Check sheet for the modelled part. Datum: model origin and axes. Units: mm. Face numbers are marked on the shaded views. A direction names the side the tool comes from. Round coordinates to 2 decimals unless told otherwise and drop trailing zeros. Order: outer loops, then holes, each group sorted by start corner. A loop starts at its lowest first (then second) coordinate and runs counter-clockwise, first axis right, second up.
```python
from build123d import *

# Parameters (mm, degrees)
BOSS_EXTRUDE1_DEPTH  = 4.5
SKETCH2_W            = 1
SKETCH2_H            = 6
BOSS_EXTRUDE2_DEPTH  = 2
SKETCH3_R            = 1
SKETCH3_R_2          = 0.5
CUT_EXTRUDE1_DEPTH   = 2
SKETCH3_2_R          = 0.5
BOSS_EXTRUDE3_DEPTH  = 2
FILLET1_R            = 1
SKETCH4_W            = 2.5
SKETCH4_H            = 2.5
CUT_EXTRUDE2_DEPTH   = 5.5000001
FILLET2_R            = 0.3
BOSS_EXTRUDE4_DEPTH  = 3.5
FILLET3_R            = 0.3
SKETCH7_W            = 0.772874032
SKETCH7_H            = 2.696512764
BOSS_EXTRUDE5_DEPTH  = 3.5
SKETCH8_W            = 0.2
SKETCH8_H            = 2
BOSS_EXTRUDE6_DEPTH  = 4
FILLET4_R            = 0.3
CUT_EXTRUDE3_DEPTH   = 0.2
FILLET4_OF_MIRROR2_R = 0.3


with BuildPart() as part:
    # Sketch1 → Boss-Extrude1 (new body)
    with BuildSketch(Plane(origin=(0, 0, 0), x_dir=(1, 0, 0), z_dir=(0, 1, 0))):
        with BuildLine():
            Line((8, -6), (8, 6))
            ThreePointArc((8, 6), (0, 10), (-8, 6))
            Line((-8, 6), (-8, -6))
            ThreePointArc((-8, -6), (0, -10), (8, -6))
        make_face()
    extrude(amount=BOSS_EXTRUDE1_DEPTH)

    # Sketch2 → Boss-Extrude2 (add)
    with BuildSketch(Plane(origin=(0, 4.5, 0), x_dir=(1, 0, 0), z_dir=(0, 1, 0))):
        with BuildLine():
            Line((4, 3), (4, -3))
            ThreePointArc((4, -3), (-5, 0), (4, 3))
        make_face()
        with Locations((-3.258806918, 0)):
            Rectangle(SKETCH2_W, SKETCH2_H, mode=Mode.SUBTRACT)
    extrude(amount=BOSS_EXTRUDE2_DEPTH)

    # Sketch3 → Cut-Extrude1 (cut)
    with BuildSketch(Plane(origin=(0, 6.5, 0), x_dir=(1, 0, 0), z_dir=(0, 1, 0))):
        Circle(SKETCH3_R)
        Circle(SKETCH3_R_2, mode=Mode.SUBTRACT)
    extrude(amount=-CUT_EXTRUDE1_DEPTH, mode=Mode.SUBTRACT)

    # Sketch3<2> → Boss-Extrude3 (add)
    with BuildSketch(Plane(origin=(0, 6.5, 0), x_dir=(1, 0, 0), z_dir=(0, 1, 0))):
        Circle(SKETCH3_2_R)
    extrude(amount=BOSS_EXTRUDE3_DEPTH)

    # Fillet1
    fillet1_edges = [part.edges().sort_by_distance(p)[0] for p in [
        (0, 4.5, 10),
        (0, 4.5, -10),
    ]]
    fillet(fillet1_edges, radius=FILLET1_R)

    # Sketch4 → Cut-Extrude2 (cut, through all)
    with BuildSketch(Plane(origin=(0, 4.5, 0), x_dir=(1, 0, 0), z_dir=(0, 1, 0))):
        with Locations((0, -10)):
            Rectangle(SKETCH4_W, SKETCH4_H)
    cut_extrude2 = extrude(amount=-CUT_EXTRUDE2_DEPTH, mode=Mode.SUBTRACT)

    # Mirror1: Cut-Extrude2 across plane
    add(cut_extrude2.mirror(Plane.XY), mode=Mode.SUBTRACT)

    # Fillet2
    fillet2_edges = [part.edges().sort_by_distance(p)[0] for p in [
        (-1.25, 2.25, -8.75),
        (1.25, 2.25, -8.75),
        (1.25, 2.25, 8.75),
        (-1.25, 2.25, 8.75),
    ]]
    fillet(fillet2_edges, radius=FILLET2_R)

    # Sketch6 → Boss-Extrude4 (add, symmetric)
    with BuildSketch(Plane.XY):
        with BuildLine():
            Line((-8, 4.5), (-8.472874032, 4.5))
            ThreePointArc((-8.472874032, 4.5), (-8.685006066, 4.412132034), (-8.772874032, 4.2))
            Line((-8.772874032, 4.2), (-8.772874032, 3.028910777))
            Line((-8.772874032, 3.028910777), (-8, 3.028910777))
            Line((-8, 3.028910777), (-8, 4.5))
        make_face()
    extrude(amount=BOSS_EXTRUDE4_DEPTH, both=True)

    # Fillet3
    fillet3_edges = [part.edges().sort_by_distance(p)[0] for p in [
        (-8, 3.764455388, -3.5),
        (-8, 3.764455388, 3.5),
    ]]
    fillet(fillet3_edges, radius=FILLET3_R)

    # Sketch7 → Boss-Extrude5 (add, symmetric)
    with BuildSketch(Plane.XY):
        with Locations((-8.386437016, 1.348256382)):
            Rectangle(SKETCH7_W, SKETCH7_H)
    extrude(amount=BOSS_EXTRUDE5_DEPTH, both=True)

    # Sketch8 → Boss-Extrude6 (add)
    with BuildSketch(Plane(origin=(0, 0, -3.5), x_dir=(-1, 0, 0), z_dir=(0, 0, -1))):
        with Locations((8.323724086, 1.346512764)):
            Rectangle(SKETCH8_W, SKETCH8_H)
    boss_extrude6 = extrude(amount=BOSS_EXTRUDE6_DEPTH)

    # Fillet4
    fillet4_edges = [part.edges().sort_by_distance(p)[0] for p in [
        (-8.323724086, 0.346512764, -7.5),
        (-8.323724086, 2.346512764, -7.5),
    ]]
    fillet(fillet4_edges, radius=FILLET4_R)

    # Sketch9 → Cut-Extrude3 (cut)
    with BuildSketch(Plane.ZY.offset(8.423724086)):
        with BuildLine():
            Line((-6.506992038, 1.790165147), (-5.08730441, 1.790165147))
            ThreePointArc((-5.08730441, 1.790165147), (-4.643652026, 1.346512764), (-5.08730441, 0.90286038))
            Line((-5.08730441, 0.90286038), (-6.506992038, 0.90286038))
            ThreePointArc((-6.506992038, 0.90286038), (-6.950644422, 1.346512764), (-6.506992038, 1.790165147))
        make_face()
    cut_extrude3 = extrude(amount=-CUT_EXTRUDE3_DEPTH, mode=Mode.SUBTRACT)

    # Mirror2: Boss-Extrude6, Cut-Extrude3 across plane
    add(boss_extrude6.mirror(Plane.XY))
    add(cut_extrude3.mirror(Plane.XY), mode=Mode.SUBTRACT)

    # Fillet4 of Mirror2
    fillet4_of_mirror2_edges = [part.edges().sort_by_distance(p)[0] for p in [
        (-8.323724086, 0.346512764, 7.5),
        (-8.323724086, 2.346512764, 7.5),
    ]]
    fillet(fillet4_of_mirror2_edges, radius=FILLET4_OF_MIRROR2_R)


solid = part.part
```
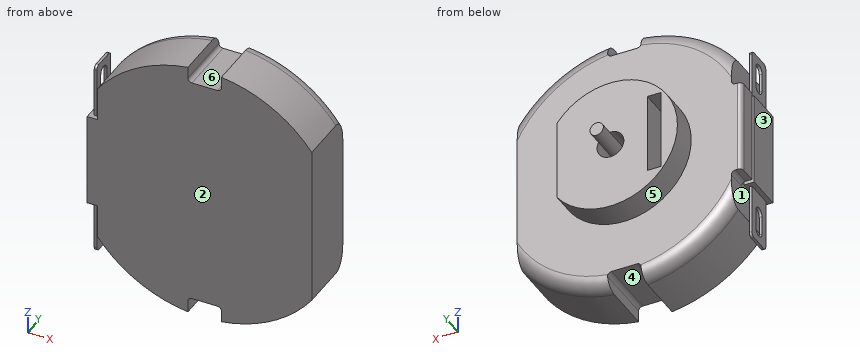
Item 1: Sectioned sample at B-B (x = 0). Record the cut outline in (y, z), and give its area (4 significant figures).
Answer:
outline: (0, -8.75) - (4.5, -8.75) - (4.5, -5) - (6.5, -5) - (6.5, -1) - (4.5, -1) - (4.5, -0.5) - (8.5, -0.5) - (8.5, 0.5) - (4.5, 0.5) - (4.5, 1) - (6.5, 1) - (6.5, 5) - (4.5, 5) - (4.5, 8.75) - (0, 8.75) - close
area: 98.75 mm2
Item 2: Release check for a two-part mould opening along Y. For the marked faces 1, 2 and 3 record: released by +Y, released by -Y, zero draft, split by the parting line, or undercut.
Answer:
face 1: undercut
face 2: released by -Y
face 3: zero draft
Item 3: Sectioned sample at C-C (z = 0). Record the cut outline in (x, y), and give its area (3 significant figures).
Answer:
outline: (-8.77, 0) - (8, 0) - (8, 4.5) - (4, 4.5) - (4, 6.5) - (1, 6.5) - (1, 4.5) - (0.5, 4.5) - (0.5, 8.5) - (-0.5, 8.5) - (-0.5, 4.5) - (-1, 4.5) - (-1, 6.5) - (-2.76, 6.5) - (-2.76, 4.5) - (-3.76, 4.5) - (-3.76, 6.5) - (-5, 6.5) - (-5, 4.5) - (-8.47, 4.5) arc R0.3 ccw to (-8.77, 4.2) - (-8.77, 3.03) - (-8, 3.03) - (-8, 2.7) - (-8.77, 2.7) - close
area: 91.2 mm2
Item 4: Go/stop test with flat-tipped pins: P1, Ø2, axis at y = 5, z = 7.5, coming from the +X side; P2, Ø2, axis at y = 2, z = 6.5, coming from the -X side; P3, Ø1.1, axis at x = -3.5, y = 5.5, coming from the +Z side. Record where each tip stops, or that it passes through.
Answer:
P1: stops at x = 6.84
P2: stops at x = -8.42
P3: stops at z = 4.04
Item 5: Scan lines: line 1 along Z through (x, y) = (0, 5.3); line 2 along X through (y, z) = (5.4, 0); line 3 along Y through (x, z) = (7, -2.75). Record each from-to range of solid material in increasing order.
Answer:
line 1: z = -5 to -1, -0.5 to 0.5, 1 to 5
line 2: x = -5 to -3.76, -2.76 to -1, -0.5 to 0.5, 1 to 4
line 3: y = 0 to 4.5
Item 6: Access from +Z, -Z, +X, -X, +Y, -Y to the whole of each face (thin tool, end or side, straight path). Record for the marked faces 4, 5 and 6.
Answer:
face 4: -Z, +Y, -Y
face 5: +Y
face 6: +Z, +Y, -Y
Item 7: Sectioned sample at A-A (y = 6). Record the cut outline in (x, z), and give its area (3 significant figures).
Answer:
outline: circle Ø1 at (0, 0); (4, -3) - (4, 3) arc R5 ccw (long way) to start; hole (-3.76, -3) - (-2.76, -3) - (-2.76, 3) - (-3.76, 3) - close; hole circle Ø2 at (0, 0)
area: 66.1 mm2
